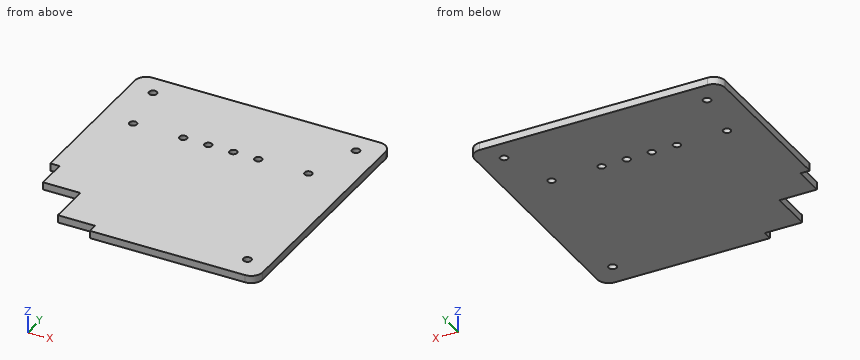
```python
from build123d import *

# Parameters (mm, degrees)
SKETCH1_W           = 127.279746886
SKETCH1_H           = 103.580209895
BOSS_EXTRUDE1_DEPTH = 3
SKETCH4_W           = 136.608236075
SKETCH4_H           = 109.831739099
CUT_EXTRUDE2_DEPTH  = 10
SKETCH5_R           = 1.55
SKETCH5_R_2         = 1.6
CUT_EXTRUDE3_DEPTH  = 10
SKETCH6_R           = 1.5
CUT_EXTRUDE4_DEPTH  = 10


with BuildPart() as part:
    # Sketch1 → Boss-Extrude1 (new body)
    with BuildSketch(Plane.XY):
        with Locations((63.639873443, 51.790104948)):
            Rectangle(SKETCH1_W, SKETCH1_H)
    extrude(amount=BOSS_EXTRUDE1_DEPTH)

    # Sketch4 → Cut-Extrude2 (cut)
    with BuildSketch(Plane.XY.offset(3)):
        with Locations((62.542352249, 51.998881619)):
            Rectangle(SKETCH4_W, SKETCH4_H)
        with BuildLine():
            Line((16.784625535, 34.613434216), (16.784625535, 97.261353998))
            add(Edge.make_bspline(
                [(16.784625535, 97.261353998), (16.814535165, 99.668332355), (18.795239635, 101.818752837), (21.284625535, 101.761353998)],
                knots=[0, 0, 0, 0, 1, 1, 1, 1], degree=3))
            Line((21.284625535, 101.761353998), (112.284625535, 101.761353998))
            add(Edge.make_bspline(
                [(112.284625535, 101.761353998), (114.750732895, 101.731954246), (116.737279379, 99.843042628), (116.784625535, 97.261353998)],
                knots=[0, 0, 0, 0, 1, 1, 1, 1], degree=3))
            Line((116.784625535, 97.261353998), (116.784625535, 6.261353998))
            add(Edge.make_bspline(
                [(116.784625535, 6.261353998), (116.776314504, 3.746141668), (114.734063303, 1.774849688), (112.284625535, 1.761353998)],
                knots=[0, 0, 0, 0, 1, 1, 1, 1], degree=3))
            Line((112.284625535, 1.761353998), (50.304591007, 1.761353998))
            Line((50.304591007, 1.761353998), (50.304591007, 5.583127479))
            Line((50.304591007, 5.583127479), (35.442949081, 5.583127479))
            Line((35.442949081, 5.583127479), (35.442949081, 22.35270073))
            Line((35.442949081, 22.35270073), (20.490844042, 22.35270073))
            Line((20.490844042, 22.35270073), (20.490844042, 34.613434216))
            Line((20.490844042, 34.613434216), (16.784625535, 34.613434216))
        make_face(mode=Mode.SUBTRACT)
    extrude(amount=-CUT_EXTRUDE2_DEPTH, mode=Mode.SUBTRACT)

    # Sketch5 → Cut-Extrude3 (cut)
    with BuildSketch(Plane.XY.offset(3)):
        with Locations((26.284625535, 93.011353998)):
            Circle(SKETCH5_R)
        with Locations((107.284625535, 93.011353998)):
            Circle(SKETCH5_R)
        with Locations((108.034625535, 11.261353998)):
            Circle(SKETCH5_R_2)
    extrude(amount=-CUT_EXTRUDE3_DEPTH, mode=Mode.SUBTRACT)

    # Sketch6 → Cut-Extrude4 (cut)
    with BuildSketch(Plane.XY.offset(3)):
        with Locations((29.784625535, 71.761353998)):
            Circle(SKETCH6_R)
        with Locations((49.784625535, 71.761353998)):
            Circle(SKETCH6_R)
        with Locations((59.784625535, 71.761353998)):
            Circle(SKETCH6_R)
        with Locations((69.784625535, 71.761353998)):
            Circle(SKETCH6_R)
        with Locations((79.784625535, 71.761353998)):
            Circle(SKETCH6_R)
        with Locations((99.784625535, 71.761353998)):
            Circle(SKETCH6_R)
    extrude(amount=-CUT_EXTRUDE4_DEPTH, mode=Mode.SUBTRACT)


solid = part.part
```
The model under review builds one solid part; all positions refer to its coordinate system, in mm. Coordinates: 2 decimals unless noted, no trailing zeros. Write each loop counter-clockwise with the first axis right and the second up, starting at its lowest first coordinate (ties: lowest second). Pieces come first, ordered by that corner, then holes. Notation, with made-up numbers: (72.5, 24.5) - (92.5, 24.5) arc R12 cw to (92.5, 39.5) - close; hole circle Ø4 at (48, -35.5). An arc over 180 degrees is marked (long way). Write item = value, one per line.
(1) Consider section B-B, the plane y = 21. Give the boundary of the cut face in (x, z).
Result sheet:
outline = (35.44, 0) - (116.78, 0) - (116.78, 3) - (35.44, 3) - close
(2) Consider section C-C, the plane x = 32.5. Give the boundary of the cut face in (y, z).
Result sheet:
outline = (22.35, 0) - (101.76, 0) - (101.76, 3) - (22.35, 3) - close
(3) For P1, Ø6, axis at x = 74.5, y = 63, coming from the -Z side; P2, Ø0.9, axis at y = 17.5, z = 2, coming from the -X side; P3, Ø0.9, axis at y = 30, z = 1.5, coming from the -X side, all flat-tipped, find the tip position at first contact; note any pin that passes through.
Result sheet:
P1 = 0
P2 = 35.44
P3 = 20.49
(4) Consider section D-D, the plane z = 1.15. State how many separate pieces and enclosed holes the cut face has, then the cut area to 3 significant figures.
Result sheet:
separate_pieces = 1
enclosed_holes = 9
area = 9,430 mm^2
(5) Consider section A-A, the plane x = 59.5. Give the boundary of the cut face in (y, z).
Result sheet:
outline = (1.76, 0) - (70.29, 0) - (70.29, 3) - (1.76, 3) - close; (73.23, 0) - (101.76, 0) - (101.76, 3) - (73.23, 3) - close
(6) For line 1 (X direction, y = 92, z = 0.7); line 2 (Y direction, x = 67.5, z = 1.85); line 3 (Y direction, x = 44.5, z = 2.45), list the stretches that pass through material, from the lowest coordinate up. Write a range as [from, to].
Result sheet:
line_1 = [16.78, 25.11], [27.46, 106.11], [108.46, 116.78]
line_2 = [1.76, 101.76]
line_3 = [5.58, 101.76]
